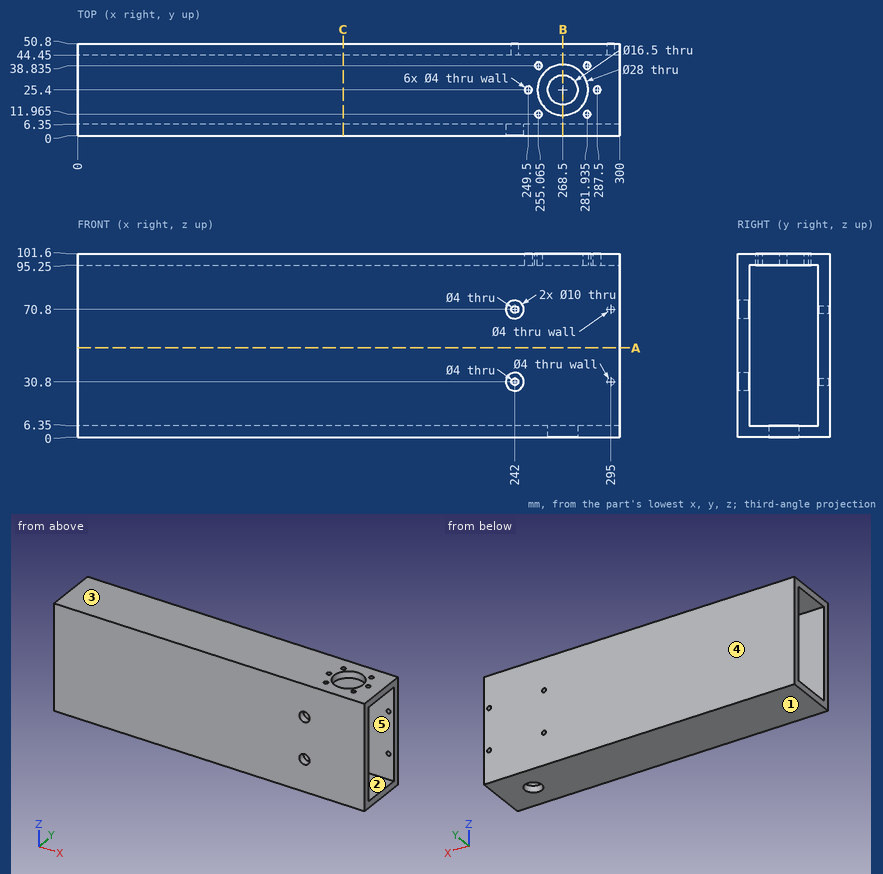
The figure shows three views and two pictorial views of one solid part (mm, origin at its lowest corner). Answer the questions. A direction names the side the tool comes from. Round coordinates to 2 decimals unless told otherwise and drop trailing zeros. Loops run counter-clockwise (first coordinate to the right, second up) from the corner with the lowest first, then second, coordinate; pieces in that order, holes last. Notation, with made-up numbers: M 43,14 L 48,14 A22 cw 48,37 Z; hole C 13,38 d2. An arc over 180 degrees is marked long. Use CSV: the item, a comma, the result in double quotes.
Q1. Section B-B, the plane x = 268.5 is taken. Determine the outline of the cut face in (y, z), then the cut area to 3 significant figures.
Determined:
outline,"M 0,0 L 17.15,0 L 17.15,6.35 L 6.35,6.35 L 6.35,95.25 L 11.4,95.25 L 11.4,101.6 L 0,101.6 Z; M 33.65,0 L 50.8,0 L 50.8,101.6 L 39.4,101.6 L 39.4,95.25 L 44.45,95.25 L 44.45,6.35 L 33.65,6.35 Z"
area,"1,490 mm2"
Q2. Consider L1, parallel to Z at x = 295, y = 49; L2, parallel to X at y = 46, z = 70.8; L3, parallel to Y at x = 67.5, z = 47.5. Determine where each line is inside the solid, lowest interval first.
Determined:
L1,"0 to 28.8, 32.8 to 68.8, 72.8 to 101.6"
L2,"0 to 240, 244 to 293, 297 to 300"
L3,"0 to 6.35, 44.45 to 50.8"
Q3. Section A-A, the plane z = 49.5 is taken. Determine the outline of the cut face in (x, y), then the cut area to 3 significant figures.
Determined:
outline,"M 0,0 L 300,0 L 300,6.35 L 0,6.35 Z; M 0,44.45 L 300,44.45 L 300,50.8 L 0,50.8 Z"
area,"3,810 mm2"
Q4. Section C-C, the plane x = 147 is taken. Determine the outline of the cut face in (y, z).
Determined:
outline,"M 0,0 L 50.8,0 L 50.8,101.6 L 0,101.6 Z; hole M 6.35,6.35 L 44.45,6.35 L 44.45,95.25 L 6.35,95.25 Z"
Q5. The mould has two halves that part along Z. Classify the marked faces 1, 2 and 3: pulls with the +Z half, pulls with the -Z half, needs draft (parallel to the pull), parting line crosses it, or undercut.
Determined:
face 1,"pulls with the -Z half"
face 2,"undercut"
face 3,"pulls with the +Z half"
Q6. A tool of negligible diameter and unlimited length cuts with its end or side. For the marked faces 4 and 5, from which of +Z, -Z, +X, -X, +Y, -Y can it reach the whole face along a straight path? Write none if from no direction.
Determined:
face 4,"+Z, -Z, +X, -X, +Y"
face 5,"+X, -X"
Q7. Each of these flat-tipped pins is pushed along its axis until it touches: pin 1 (4 mm diameter, centred on y = 7.5, z = 87.5, fed in from -X); pin 2 (21.5 mm diameter, centred on x = 268.5, y = 25.4, fed in from +Z); pin 3 (3.5 mm diameter, centred on x = 242, z = 70.8, fed in from +Y); pin 4 (8 mm diameter, centred on x = 242, z = 30.8, fed in from -Y). Where does it stop, or does it pass through?
Determined:
pin 1,"x = 0"
pin 2,"z = 6.35"
pin 3,"through"
pin 4,"y = 44.45"
